from build123d import *

# Parameters (mm, degrees)
SKETCH1_R           = 1
BOSS_EXTRUDE1_DEPTH = 25
CUT_EXTRUDE1_START  = -20.1
SKETCH2_R           = 2.5
CUT_EXTRUDE1_DEPTH  = 15.2
BOSS_EXTRUDE2_START = -4.9
BOSS_EXTRUDE2_DEPTH = 4.9


with BuildPart() as part:
    # Sketch1 → Boss-Extrude1 (new body)
    with BuildSketch(Plane.XY):
        with BuildLine():
            Line((-3, -1.5), (3, -1.5))
            ThreePointArc((3, -1.5), (4.132206562, 1.085942892), (6.800319489, 2.00798722))
            ThreePointArc((6.800319489, 2.00798722), (8.837008612, 6.195700257), (4.5, 4.5))
            ThreePointArc((4.5, 4.5), (3.621320344, 2.378679656), (1.5, 1.5))
            Line((1.5, 1.5), (-3, 1.5))
            Line((-3, 1.5), (-3, -1.5))
        make_face()
        with Locations((7, 4.5)):
            Circle(SKETCH1_R, mode=Mode.SUBTRACT)
    extrude(amount=BOSS_EXTRUDE1_DEPTH)

    # Sketch2 → Cut-Extrude1 (cut)
    with BuildSketch(Plane.XY.offset(25).offset(CUT_EXTRUDE1_START)):
        with Locations((7, 4.5)):
            Circle(SKETCH2_R)
    extrude(amount=CUT_EXTRUDE1_DEPTH, mode=Mode.SUBTRACT)

    # Sketch4 → Boss-Extrude2 (add)
    with BuildSketch(Plane.XY.offset(25).offset(BOSS_EXTRUDE2_START)):
        with BuildLine():
            Line((3, -1.5), (9.5, -1.5))
            Line((9.5, -1.5), (9.5, 4.5))
            ThreePointArc((9.5, 4.5), (8.695700257, 2.662991388), (6.800319489, 2.00798722))
            ThreePointArc((6.800319489, 2.00798722), (4.132206562, 1.085942892), (3, -1.5))
        make_face()
    extrude(amount=BOSS_EXTRUDE2_DEPTH)


solid = part.part
The listing builds one solid part. Answer for the finished solid, in the listing's coordinates (mm). A direction names the side the tool comes from. Give positions to 0.01 mm unless a question says otherwise; leave off trailing zeros. Loops run counter-clockwise (first coordinate to the right, second up) from the corner with the lowest first, then second, coordinate; pieces in that order, holes last. Notation, with made-up numbers: (14, 71.25) - (27, 71.25) arc R11 cw to (27, 90.25) - close; hole circle Ø7 at (49.25, 59.5). An arc over 180 degrees is marked (long way). Use one line per item in the form item = value.
1. Find the intervals of material crossed by line 1 along X through (y, z) = (4.5, 2.75); line 2 along Y through (x, z) = (7, 3.4); line 3 along Y through (x, z) = (7, 22.8), in increasing order. Write a range as [from, to].
Calculated:
line_1 = [4.5, 6], [8, 9.5]
line_2 = [2, 3.5], [5.5, 7]
line_3 = [-1.5, 3.5], [5.5, 7]
2. Section C-C on z = 21.5 is taken. Give the vertices of the cut face in (x, y).
Calculated:
outline = (-3, -1.5) - (9.5, -1.5) - (9.5, 4.5) arc R2.5 ccw to (4.5, 4.5) arc R3 cw to (1.5, 1.5) - (-3, 1.5) - close; hole circle Ø2 at (7, 4.5)
3. Section D-D on y = 0.5 is taken. Give the vertices of the cut face in (x, z).
Calculated:
outline = (-3, 0) - (3.62, 0) - (3.62, 20.1) - (9.5, 20.1) - (9.5, 25) - (-3, 25) - close
4. Section A-A on z = 4.5 is taken. Give the vertices of the cut face in (x, y), then the cut area to 3 significant figures.
Calculated:
outline = (-3, -1.5) - (3, -1.5) arc R3.52 cw to (6.8, 2.01) arc R2.5 ccw (long way) to (4.5, 4.5) arc R3 cw to (1.5, 1.5) - (-3, 1.5) - close; hole circle Ø2 at (7, 4.5)
area = 39.6 mm^2
5. Section B-B on x = 8.25 is taken. Give the vertices of the cut face in (y, z).
Calculated:
outline = (-1.5, 20.1) - (6.67, 20.1) - (6.67, 25) - (-1.5, 25) - close; (2.33, 0) - (6.67, 0) - (6.67, 4.9) - (2.33, 4.9) - close
6. Given pin 1 Ø5 at (x, z) = (6.5, 12) entering from -Y; pin 2 Ø3 at (y, z) = (4.5, 14.5) entering from -X; pin 3 Ø3.5 at (x, z) = (-0.5, 13) entering from +Y, each flat-ended and moving along its own axis, determine where each tip first touches the part or whether it passes through.
Calculated:
pin_1 = 0.96
pin_2 = 4.1
pin_3 = 1.5
7. Which of the six approach directions +Z, -Z, +X, -X, +Y, -Y give full straight-line access (tool end or side, diameter ignored) to faces 1 (the face through (-1, 1.5, 12)), 2 (the face through (7, 2, 20.1)), 3 (the face through (5, 3, 12))?
Calculated:
face_1 = +Z, -Z, -X, +Y
face_2 = +X
face_3 = +X, +Y
8. The mould has two halves that part along Y. Classify faces 4 (the face through (9, 6, 2)), 5 (the face through (6.263, 5.176, 2.416)), 6 (the face through (5, 2, 0)): pulls with the +Y half, pulls with the -Y half, needs draft (parallel to the pull), parting line crosses it, or undercut.
Calculated:
face_4 = parting line crosses it
face_5 = undercut
face_6 = needs draft
